Could you check a few things on this model? Use its own coordinates, in mm. A direction names the side the tool comes from. Coordinates: 2 decimals unless noted, no trailing zeros. Order: outer loops, then holes, each group sorted by start corner. A loop starts at its lowest first (then second) coordinate and runs counter-clockwise, first axis right, second up. Notation, with made-up numbers: M -22,69.5 L -6,69.5 A22 cw -6,97.5 Z; hole C 17,62.25 d7. An arc over 180 degrees is marked long. Put each result on its own line as item: value. Start each with the question number.
```python
from build123d import *

# Parameters (mm, degrees)
F0_R     = 5
F0_R_2   = 7.25
F1_DEPTH = 12.7
F2_DEPTH = 2


with BuildPart() as f1:
    # F0 (on Top) → F1 (new body)
    with BuildSketch(Plane.XY):
        with BuildLine():
            Line((8.5, 0), (8.5, 16.5))
            ThreePointArc((8.5, 16.5), (3.596169, 24.20179), (-5.457075, 23.016927))
            Line((-5.457075, 23.016927), (-6.578885, 21.882218))
            Line((-6.578885, 21.882218), (-15.885772, 12.46832))
            ThreePointArc((-15.885772, 12.46832), (-17.61895, 8.249909), (-15.885645, 4.03155))
            Line((-15.885645, 4.03155), (-6.581584, -5.378917))
            Line((-6.581584, -5.378917), (-5.45341, -6.519994))
            ThreePointArc((-5.45341, -6.519994), (3.598334, -7.700779), (8.5, 0))
        make_face()
        with Locations((-11.61895, 8.25)):
            Circle(F0_R, mode=Mode.SUBTRACT)
        Circle(F0_R_2, mode=Mode.SUBTRACT)
        with Locations((0, 16.5)):
            Circle(F0_R_2, mode=Mode.SUBTRACT)
    extrude(amount=F1_DEPTH)

    # F0 (on Top) → F2 (join)
    with BuildSketch(Plane.XY):
        with BuildLine():
            Line((8.5, 0), (8.5, 16.5))
            ThreePointArc((8.5, 16.5), (3.596169, 24.20179), (-5.457075, 23.016927))
            Line((-5.457075, 23.016927), (-6.578885, 21.882218))
            Line((-6.578885, 21.882218), (-15.885772, 12.46832))
            ThreePointArc((-15.885772, 12.46832), (-17.61895, 8.249909), (-15.885645, 4.03155))
            Line((-15.885645, 4.03155), (-6.581584, -5.378917))
            Line((-6.581584, -5.378917), (-5.45341, -6.519994))
            ThreePointArc((-5.45341, -6.519994), (3.598334, -7.700779), (8.5, 0))
        make_face()
        with Locations((-11.61895, 8.25)):
            Circle(F0_R, mode=Mode.SUBTRACT)
        Circle(F0_R_2, mode=Mode.SUBTRACT)
        with Locations((0, 16.5)):
            Circle(F0_R_2, mode=Mode.SUBTRACT)
        with Locations((0, 16.5)):
            Circle(F0_R_2)
        Circle(F0_R_2)
        with Locations((-11.61895, 8.25)):
            Circle(F0_R)
    extrude(amount=F2_DEPTH)


solid = f1.part
```
Item 1: If we section it at A-A on z = 8.5: Write out the boundary of the cut face in (x, y), then the cut area to 3 significant figures.
Item 2: I need wall thicknesses on probe 1 along Y at (x, z) = (0, 8.75); probe 2 along X at (y, z) = (8.5, 3.5); probe 3 along X at (y, z) = (4, 6.25). Which ranges of each line are inside material? Lowest first, please.
Item 3: For pin 1 Ø3 at (x, z) = (4.5, 11) entering from +Y; pin 2 Ø2 at (x, z) = (-5, 5.5) entering from +Y; pin 3 Ø7 at (x, y) = (-1, 20) entering from +Z, each with a flat end and sliding along its axis, tell me the tip position at first contact or that it passes through.
Item 4: For faces 1 (the flat face through (8.5, 8, 6)), 2 (the cylindrical face through (3.35, -6.43, 7.28)), which set-ups out of +Z, -Z, +X, -X, +Y, -Y let a thin tool reach every point of the face, with its end or its side?
Item 5: If we section it at B-B on y = 8.25: Write out the boundary of the cut face in (x, z), then the cut area to 3 significant figures.
Item 6: If we mould it in two halves opening along X, with no side actions, what happens to faces 3 (the cylindrical face through (-17.62, 8.32, 6.26)), 4 (the cylindrical face through (-8.931, 12.466, 7.275)), 5 (the flat face through (-2, 8, 0))? For each: released by +X, released by -X, zero draft, split by the parting line, or undercut.
Item 7: If we section it at C-C on x = 0: Write out the boundary of the cut face in (y, z).
Item 8: If we section it at D-D on y = -2: Write out the boundary of the cut face in (x, z).
Geometry check:
1. outline: M -15.89,4.03 L -6.58,-5.38 L -5.45,-6.52 A8.5 ccw 8.5,0 L 8.5,16.5 A8.5 ccw -5.46,23.02 L -6.58,21.88 L -15.89,12.47 A6 ccw Z; hole C -11.62,8.25 d10; hole C 0,0 d14.5; hole C 0,16.5 d14.5
1. area: 229 mm²
2. probe 1: y = -8.5 to -7.25, 7.25 to 9.25, 23.75 to 25
2. probe 2: x = -17.61 to -16.61, -6.63 to 8.5
2. probe 3: x = -15.85 to -14.25, -8.99 to -6.05, 6.05 to 8.5
3. pin 1: stops at y = 24.45
3. pin 2: stops at y = 24
3. pin 3: stops at z = 2
4. face 1: +Z, -Z, +X, +Y, -Y
4. face 2: +Z
5. outline: M -17.62,0 L 8.5,0 L 8.5,12.7 L -6.62,12.7 L -6.62,2 L -16.62,2 L -16.62,12.7 L -17.62,12.7 Z
5. area: 225 mm²
6. face 3: released by -X
6. face 4: undercut
6. face 5: zero draft
7. outline: M -8.5,0 L 25,0 L 25,12.7 L 23.75,12.7 L 23.75,2 L 9.25,2 L 9.25,12.7 L 7.25,12.7 L 7.25,2 L -7.25,2 L -7.25,12.7 L -8.5,12.7 Z
8. outline: M -9.92,0 L 8.26,0 L 8.26,12.7 L 6.97,12.7 L 6.97,2 L -6.97,2 L -6.97,12.7 L -9.92,12.7 Z
